from build123d import *

# Parameters (mm, degrees)
F0_W     = 85
F0_H     = 50
F1_DEPTH = 10
F4_SIZE  = 2.54
F2_R     = 1.830609
F2_R_2   = 1.251164
F3_R     = 2.466277
F3_R_2   = 5.012631
F3_R_3   = 3.402789
F5_DEPTH = 5


with BuildPart() as f1:
    # F0 (on Top) → F1 (new body)
    with BuildSketch(Plane.XY):
        with Locations((13.320725, 22.314699)):
            Rectangle(F0_W, F0_H)
    extrude(amount=F1_DEPTH)

    # F4
    f4_edges = [f1.edges().sort_by_distance(p)[0] for p in [
        (13.320725, 47.314699, 10),
        (-29.179275, 22.314699, 10),
        (13.320725, -2.685301, 10),
        (55.820725, 22.314699, 10),
    ]]
    chamfer(f4_edges, length=F4_SIZE)

    # F2 (on face) + F3 (on face) → F5 (cut)
    with BuildSketch(Plane.XY.offset(10)):
        Polygon((-21.920681, 42.516656), (-26.938394, 25.330184), (-24.203247, 25.330184), (-21.920681, 31.555358), (-18.619085, 31.555358), (-16.336523, 25.330184), (-12.91264, 25.330184), (-18.619085, 42.516656), align=None)
        Polygon((-20.203851, 39.413154), (-18.619085, 34.790922), (-21.920681, 34.790922), align=None, mode=Mode.SUBTRACT)
        with BuildLine():
            ThreePointArc((-5.676832, 31.621389), (-11.941997, 28.947097), (-5.676832, 26.272805))
            Line((-5.676832, 26.272805), (-5.676832, 25.018198))
            Line((-5.676832, 25.018198), (-3.56381, 25.018198))
            Line((-3.56381, 25.018198), (-3.56381, 40.931888))
            Line((-3.56381, 40.931888), (-5.676832, 40.931888))
            Line((-5.676832, 40.931888), (-5.676832, 31.621389))
        make_face()
        with Locations((-8.245731, 29.008828)):
            Circle(F2_R, mode=Mode.SUBTRACT)
        with BuildLine():
            Line((-1.252693, 32.6779), (-1.252693, 24.886135))
            Line((-1.252693, 24.886135), (0.794296, 24.886135))
            Line((0.794296, 24.886135), (0.794296, 28.517889))
            ThreePointArc((0.794296, 28.517889), (3.322981, 31.046574), (5.851666, 28.517889))
            Line((5.851666, 28.517889), (7.805725, 28.537814))
            ThreePointArc((7.805725, 28.537814), (5.231823, 32.219617), (0.794296, 31.520326))
            Line((0.794296, 31.520326), (0.794296, 32.6779))
            Line((0.794296, 32.6779), (-1.252693, 32.6779))
        make_face()
        Polygon((10.287394, 31.555358), (8.628487, 31.555358), (8.628487, 24.886135), (10.287394, 24.851044), align=None)
        with Locations((9.245559, 35.428446)):
            Circle(F2_R_2)
        with BuildLine():
            Line((15.827652, 31.931706), (15.519116, 30.183338))
            ThreePointArc((15.519116, 30.183338), (11.282193, 27.115575), (15.827652, 24.526851))
            Line((15.827652, 24.526851), (15.827652, 23.395553))
            Line((15.827652, 23.395553), (17.37033, 23.395553))
            Line((17.37033, 23.395553), (17.37033, 31.931706))
            Line((17.37033, 31.931706), (15.827652, 31.931706))
        make_face()
        with BuildLine():
            ThreePointArc((15.416271, 25.658149), (13.135805, 27.425758), (15.519116, 29.05204))
            Line((15.519116, 29.05204), (15.416271, 25.658149))
        make_face(mode=Mode.SUBTRACT)
        with BuildLine():
            Line((21.175602, 31.931706), (19.94146, 31.931706))
            Line((19.94146, 31.931706), (19.94146, 24.526851))
            Line((19.94146, 24.526851), (21.175602, 24.526851))
            Line((21.175602, 24.526851), (21.175602, 28.84635))
            ThreePointArc((21.175602, 28.84635), (22.746854, 31.009158), (25.289411, 30.183338))
            Line((25.289411, 30.183338), (25.289411, 24.526851))
            Line((25.289411, 24.526851), (26.523555, 24.526851))
            Line((26.523555, 24.526851), (26.523555, 30.286184))
            ThreePointArc((26.523555, 30.286184), (24.083285, 32.382249), (21.175602, 31.0061))
            Line((21.175602, 31.0061), (21.175602, 31.931706))
        make_face()
    with BuildSketch(Plane.XY.offset(10)):
        with BuildLine():
            Line((-15.212267, 17.637189), (-13.020429, 17.527597))
            ThreePointArc((-13.020429, 17.527597), (-23.456448, 22.38112), (-19.705536, 11.500043))
            ThreePointArc((-19.705536, 11.500043), (-15.363439, 5.240268), (-22.77411, 7.006774))
            Line((-22.77411, 7.006774), (-24.746763, 6.677999))
            ThreePointArc((-24.746763, 6.677999), (-13.507007, 4.069267), (-19.705536, 13.801472))
            ThreePointArc((-19.705536, 13.801472), (-21.949485, 20.979729), (-15.212267, 17.637189))
        make_face()
        Polygon((-9.757687, 12.376778), (-12.034101, 12.376778), (-8.198384, 2.294322), (-5.896954, 2.294322), (-3.705117, 9.417796), (0, 2.294322), (2.103255, 2.294322), (6.377339, 12.376778), (3.966318, 12.376778), (1.226519, 5.253303), (-2.478598, 12.376778), (-5.020219, 12.376778), (-7.047669, 5.253303), align=None)
        with BuildLine():
            Line((15.0351, 2.294322), (15.0351, 12.376778))
            Line((15.0351, 12.376778), (12.952854, 12.376778))
            Line((12.952854, 12.376778), (12.952854, 10.842491))
            ThreePointArc((12.952854, 10.842491), (5.970738, 7.280754), (12.952854, 3.719016))
            Line((12.952854, 3.719016), (12.952854, 2.294322))
            Line((12.952854, 2.294322), (15.0351, 2.294322))
        make_face()
        with Locations((10.370258, 7.280754)):
            Circle(F3_R, mode=Mode.SUBTRACT)
        with BuildLine():
            Line((19.199593, 12.376778), (17.226938, 12.376778))
            Line((17.226938, 12.376778), (17.226938, 2.030088))
            Line((17.226938, 2.030088), (19.199593, 2.030088))
            Line((19.199593, 2.030088), (19.199593, 8.450842))
            ThreePointArc((19.199593, 8.450842), (21.691911, 9.686684), (24.021637, 8.166376))
            Line((24.021637, 8.166376), (24.021637, 2.030088))
            Line((24.021637, 2.030088), (25.764035, 2.030088))
            Line((25.764035, 2.030088), (25.764035, 8.450842))
            ThreePointArc((25.764035, 8.450842), (23.066805, 11.626978), (19.199593, 10.075347))
            Line((19.199593, 10.075347), (19.199593, 12.376778))
        make_face()
        with BuildLine():
            Line((32.3296, 8.760245), (33.227358, 8.760245))
            ThreePointArc((33.227358, 8.760245), (28.437176, 9.918983), (31.145109, 5.801263))
            ThreePointArc((31.145109, 5.801263), (32.104813, 3.227295), (29.444952, 3.913939))
            Line((29.444952, 3.913939), (28.267544, 3.913939))
            ThreePointArc((28.267544, 3.913939), (32.81246, 2.257757), (31.145109, 6.798588))
            ThreePointArc((31.145109, 6.798588), (29.156537, 9.33777), (32.3296, 8.760245))
        make_face()
        with Locations((38.923081, 6.327625)):
            Circle(F3_R_2)
        with Locations((38.923081, 6.327625)):
            Circle(F3_R_3, mode=Mode.SUBTRACT)
        with BuildLine():
            Line((45.981784, 1.907284), (47.400411, 2.030088))
            Line((47.400411, 2.030088), (47.400411, 8.450842))
            ThreePointArc((47.400411, 8.450842), (49.325353, 9.178813), (51.250294, 8.450842))
            Line((51.250294, 8.450842), (51.250294, 2.030088))
            Line((51.250294, 2.030088), (52.535262, 2.141321))
            Line((52.535262, 2.141321), (52.535262, 8.450842))
            ThreePointArc((52.535262, 8.450842), (50.256526, 10.269882), (47.400411, 9.683236))
            Line((47.400411, 9.683236), (47.400411, 11.202979))
            Line((47.400411, 11.202979), (45.981784, 11.226063))
            Line((45.981784, 11.226063), (45.981784, 1.907284))
        make_face()
    extrude(amount=-F5_DEPTH, mode=Mode.SUBTRACT)


solid = f1.part
Input: part model. Units: mm. Frame: model coordinates. A direction names the side the tool comes from. Give positions to 0.01 mm unless a question says otherwise; leave off trailing zeros. Write each loop counter-clockwise with the first axis right and the second up, starting at its lowest first coordinate (ties: lowest second). Pieces come first, ordered by that corner, then holes. Notation, with made-up numbers: M -1.5,72.5 L 52.5,72.5 A27 cw 52.5,98.5 Z; hole C 62,39.5 d9. An arc over 180 degrees is marked long. Write item = value, one per line. Start each with the question number.
1) Reachability of faces 1 (the flat face through (12.726, -1.398, 8.748)), 2 (the flat face through (-7, 2.294, 8)) from +Z, -Z, +X, -X, +Y, -Y: full face, straight path, thin tool, end or side. Return the list, or none.
2) Material intervals for line 1 along Y through (x, z) = (20.5, 8); line 2 along X through (y, z) = (37, 5.5); line 3 along Z through (x, y) = (2.5, 31), sorted ascending. Write a range as [from, to].
3) Cut plane B-B on x = -11. Return the cut outline in (y, z).
4) Cut plane D-D on x = 14. Return the cut outline in (y, z).
5) Cut plane A-A on y = 15.5. Return the cut outline in (x, z), then the cut area to 3 significant figures.
6) First-contact query: pin 1 Ø0.5 at (x, z) = (16, 8) entering from +Y; pin 2 Ø0.7 at (y, z) = (3, 8) entering from +X; pin 3 Ø0.8 at (x, y) = (9.5, 36) entering from +Z. Flat tips, straight axial feed; report the tip coordinate or a pass-through.
7) Cut plane C-C on z = 8.5. Count the separate pieces of the cut face and the enclosed holes in it, then the cut area to 3 significant figures.
Solved:
q1.face_1 = +Z, +X, -X, -Y
q1.face_2 = +Z
q2.line_1 = [-2.15, 9.5], [11.29, 24.53], [31.93, 46.77]
q2.line_2 = [-29.18, -23.53], [-21.1, -19.38], [-16.79, -5.68], [-3.56, 55.82]
q2.line_3 = [0, 5]
q3.outline = M -2.69,0 L 47.31,0 L 47.31,7.46 L 44.77,10 L 31.41,10 L 31.41,5 L 26.48,5 L 26.48,10 L 12.38,10 L 12.38,5 L 9.66,5 L 9.66,10 L -0.15,10 L -2.69,7.46 Z
q4.outline = M -2.69,0 L 47.31,0 L 47.31,7.46 L 44.77,10 L 30.37,10 L 30.37,5 L 28.9,5 L 28.9,10 L 25.84,10 L 25.84,5 L 24.2,5 L 24.2,10 L 12.38,10 L 12.38,5 L 2.29,5 L 2.29,10 L -0.15,10 L -2.69,7.46 Z
q5.outline = M -29.18,0 L 55.82,0 L 55.82,7.46 L 53.28,10 L -22.63,10 L -22.63,5 L -25.11,5 L -25.11,10 L -26.64,10 L -29.18,7.46 Z
q5.area = 831 mm2
q6.pin_1 = 47.02
q6.pin_2 = 55.63
q6.pin_3 = 5
q7.separate_pieces = 6
q7.enclosed_holes = 14
q7.area = 3,330 mm2
